from build123d import *

# Parameters (mm, degrees)
F0_W     = 2438.4
F0_H     = 88.9
F1_DEPTH = 38.1
F2_W     = 38.1
F2_H     = 88.9
F3_DEPTH = 1143
F4_W     = 2438.4
F4_H     = 38.1
F5_DEPTH = 88.9


with BuildPart() as f1:
    # F0 (on Top) → F1 (new body)
    with BuildSketch(Plane.XY):
        Rectangle(F0_W, F0_H)
    extrude(amount=F1_DEPTH)

    # F2 (on face) → F3 (join)
    with BuildSketch(Plane.XY.offset(38.1)):
        with Locations((1200.15, 0)):
            Rectangle(F2_W, F2_H)
        with Locations((882.65, 0)):
            Rectangle(F2_W, F2_H)
        with Locations((476.25, 0)):
            Rectangle(F2_W, F2_H)
        with Locations((69.85, 0)):
            Rectangle(F2_W, F2_H)
        with Locations((-336.55, 0)):
            Rectangle(F2_W, F2_H)
        with Locations((-742.95, 0)):
            Rectangle(F2_W, F2_H)
        with Locations((-1200.15, 0)):
            Rectangle(F2_W, F2_H)
        with Locations((-1162.05, 0)):
            Rectangle(F2_W, F2_H)
    extrude(amount=F3_DEPTH)

    # F4 (on face) → F5 (join)
    with BuildSketch(Plane.XZ.offset(44.45)):
        with Locations((0, 1200.15)):
            Rectangle(F4_W, F4_H)
    extrude(amount=-F5_DEPTH)


solid = f1.part
Check sheet for the modelled part. Datum: model origin and axes. Units: mm. A direction names the side the tool comes from. Round coordinates to 2 decimals unless told otherwise and drop trailing zeros. Loops run counter-clockwise (first coordinate to the right, second up) from the corner with the lowest first, then second, coordinate; pieces in that order, holes last. Notation, with made-up numbers: M 29.25,43 L 37.25,43 A29 ccw 37.25,70 Z; hole C 21.25,85 d6. An arc over 180 degrees is marked long. One line per item, written item: value.
(1) Sectioned sample at A-A, the plane y = 25. Record the cut outline in (x, z), then the cut area to 3 significant figures.
Computed values:
outline: M -1219.2,0 L 1219.2,0 L 1219.2,1219.2 L -1219.2,1219.2 Z; hole M -1143,38.1 L -762,38.1 L -762,1181.1 L -1143,1181.1 Z; hole M -723.9,38.1 L -355.6,38.1 L -355.6,1181.1 L -723.9,1181.1 Z; hole M -317.5,38.1 L 50.8,38.1 L 50.8,1181.1 L -317.5,1181.1 Z; hole M 88.9,38.1 L 457.2,38.1 L 457.2,1181.1 L 88.9,1181.1 Z; hole M 495.3,38.1 L 863.6,38.1 L 863.6,1181.1 L 495.3,1181.1 Z; hole M 901.7,38.1 L 1181.1,38.1 L 1181.1,1181.1 L 901.7,1181.1 Z
area: 534,000 mm^2
(2) Release check for a two-part mould opening along X. For faces 3 (the face through (-1219.2, -1, 601)), 4 (the face through (85, 44.45, 658)), 5 (the face through (901.7, -1, 602)) record: +X half, -X half, draft (parallel to the pull), parting line (faces both ways), or undercut.
Computed values:
face 3: -X half
face 4: draft
face 5: undercut
(3) Thickness scan on line 1 (Z direction, x = -368.5, y = -31). Record the ranges inside material, lowest first.
Computed values:
line 1: z = 0 to 38.1, 1181.1 to 1219.2
(4) Sectioned sample at C-C, the plane x = -960.5. Record the cut outline in (y, z).
Computed values:
outline: M -44.45,0 L 44.45,0 L 44.45,38.1 L -44.45,38.1 Z; M -44.45,1181.1 L 44.45,1181.1 L 44.45,1219.2 L -44.45,1219.2 Z
(5) Sectioned sample at B-B, the plane z = 302. Record the cut outline in (x, y), then the cut area to 3 significant figures.
Computed values:
outline: M -1219.2,-44.45 L -1143,-44.45 L -1143,44.45 L -1219.2,44.45 Z; M -762,-44.45 L -723.9,-44.45 L -723.9,44.45 L -762,44.45 Z; M -355.6,-44.45 L -317.5,-44.45 L -317.5,44.45 L -355.6,44.45 Z; M 50.8,-44.45 L 88.9,-44.45 L 88.9,44.45 L 50.8,44.45 Z; M 457.2,-44.45 L 495.3,-44.45 L 495.3,44.45 L 457.2,44.45 Z; M 863.6,-44.45 L 901.7,-44.45 L 901.7,44.45 L 863.6,44.45 Z; M 1181.1,-44.45 L 1219.2,-44.45 L 1219.2,44.45 L 1181.1,44.45 Z
area: 27,100 mm^2
(6) Access from +Z, -Z, +X, -X, +Y, -Y to the whole of each face (thin tool, end or side, straight path). Record for faces 1 (the face through (85, -44.45, 658)), 2 (the face through (-136, -1, 1181.1)).
Computed values:
face 1: +Z, -Z, +X, -X, -Y
face 2: +Y, -Y
